Source: CAD feature listing. Evaluate the final solid. Frame: model axes, mm. Give positions to 0.01 mm unless a question says otherwise; leave off trailing zeros. Order: outer loops, then holes, each group sorted by start corner. A loop starts at its lowest first (then second) coordinate and runs counter-clockwise, first axis right, second up. Notation, with made-up numbers: M 49.25,-22 L 93.25,-22 A19 ccw 93.25,1 Z; hole C 14,73.5 d11. An arc over 180 degrees is marked long. Use CSV: the item, a comma, the result in double quotes. Start each with the question number.
1. Section query B-B, the plane x = 1.5. Return the cut outline in (y, z).
2. Section query A-A, the plane z = 21. Return the cut outline in (x, y).
3. Line query: line 1 along X through (y, z) = (2.1, 45); line 2 along Z through (x, y) = (-12, 2.05); line 3 along Z through (x, y) = (-5, 2.65). Output: solid intervals per line, ascending. Write a range as [from, to].
4. Section query D-D, the plane x = -4.2. Return the cut outline in (y, z).
5. Section query C-C, the plane y = 2.3. Return the cut outline in (x, z), plus the area to 3 significant figures.
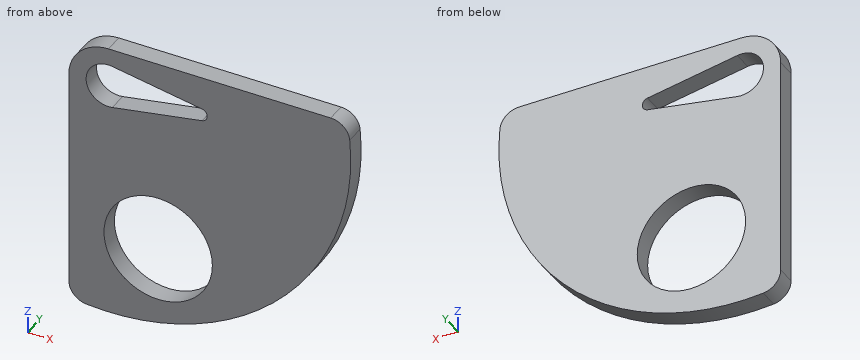
from build123d import *

# Parameters (mm, degrees)
SKETCH8_R           = 1.5
SKETCH8_R_2         = 8.5
BOSS_EXTRUDE3_DEPTH = 3
CUT_EXTRUDE3_DEPTH  = 4
FILLET1_R           = 3


with BuildPart() as part:
    # Sketch8 → Boss-Extrude3 (new body)
    with BuildSketch(Plane(origin=(0, 0, 0), x_dir=(1, 0, 0), z_dir=(0, 1, 0))):
        with BuildLine():
            Line((-12, -51.2), (25.490798871, -51.2))
            ThreePointArc((25.490798871, -51.2), (14.870057685, -18.129942315), (-18.2, -7.509201129))
            Line((-18.2, -7.509201129), (-18.2, -45))
            ThreePointArc((-18.2, -45), (-16.384062043, -49.384062043), (-12, -51.2))
        make_face()
        with Locations((-12, -45)):
            Circle(SKETCH8_R, mode=Mode.SUBTRACT)
        with Locations((-4.2, -20.197580763)):
            Circle(SKETCH8_R_2, mode=Mode.SUBTRACT)
    extrude(amount=BOSS_EXTRUDE3_DEPTH)

    # Sketch10 → Cut-Extrude3 (cut, through all)
    with BuildSketch(Plane(origin=(0, 0, 0), x_dir=(1, 0, 0), z_dir=(0, 1, 0))):
        with BuildLine():
            Line((-11.396551724, -41.552413862), (2.672413793, -44.014975389))
            ThreePointArc((2.672413793, -44.014975389), (3.5, -45), (2.672413793, -45.985024611))
            Line((2.672413793, -45.985024611), (-11.396551724, -48.447586138))
            ThreePointArc((-11.396551724, -48.447586138), (-15.5, -45), (-11.396551724, -41.552413862))
        make_face()
    extrude(amount=CUT_EXTRUDE3_DEPTH, mode=Mode.SUBTRACT)

    # Fillet1
    fillet1_edges = [part.edges().sort_by_distance(p)[0] for p in [
        (-18.2, 1.5, 7.509201129),
        (25.490798871, 1.5, 51.2),
    ]]
    fillet(fillet1_edges, radius=FILLET1_R)


solid = part.part
Result set:
1,outline,"M 0,9.48 L 3,9.48 L 3,13.89 L 0,13.89 Z; M 0,26.5 L 3,26.5 L 3,43.81 L 0,43.81 Z; M 0,46.19 L 3,46.19 L 3,51.2 L 0,51.2 Z"
2,outline,"M -18.2,0 L -12.66,0 L -12.66,3 L -18.2,3 Z; M 4.26,0 L 17.46,0 L 17.46,3 L 4.26,3 Z"
3,line 1,"[-18.2, -15.5], [3.5, 26]"
3,line 2,"[7, 16.82], [23.58, 41.5], [48.5, 51.2]"
3,line 3,"[7.65, 11.74], [28.66, 42.67], [47.33, 51.2]"
4,outline,"M 0,7.81 L 3,7.81 L 3,11.7 L 0,11.7 Z; M 0,28.7 L 3,28.7 L 3,42.81 L 0,42.81 Z; M 0,47.19 L 3,47.19 L 3,51.2 L 0,51.2 Z"
5,outline,"M -18.2,10.15 A3 ccw -15.47,7.16 A38 ccw 25.84,48.47 A3 ccw 22.85,51.2 L -12,51.2 A6.2 ccw -18.2,45 Z; hole C -4.2,20.2 d17; hole M -11.4,41.55 L 2.67,44.01 A1 ccw 2.67,45.99 L -11.4,48.45 A3.5 ccw long Z"
5,area,"1,320 mm2"
